Verification items for the finished model (mm, model axes). A direction names the side the tool comes from. Round coordinates to 2 decimals unless told otherwise and drop trailing zeros. Write each loop counter-clockwise with the first axis right and the second up, starting at its lowest first coordinate (ties: lowest second). Pieces come first, ordered by that corner, then holes. Notation, with made-up numbers: (78, -18.5) - (104, -18.5) arc R30 ccw to (104, 16.5) - close; hole circle Ø4 at (-26, 62.25). An arc over 180 degrees is marked (long way). Answer as a JSON object with one key per item and string values.
```python
from build123d import *

# Parameters (mm, degrees)
SKETCH1_W           = 144.53
SKETCH1_H           = 37.629508446
SKETCH1_R           = 1.6
BOSS_EXTRUDE1_DEPTH = 5


with BuildPart() as part:
    # Sketch1 → Boss-Extrude1 (new body)
    # profile 1 of 2: a face of its own
    with BuildSketch(Plane(origin=(0, 0, 0), x_dir=(1, 0, 0), z_dir=(0, 1, 0))):
        with Locations((-90.246144653, 26.488873013)):
            Rectangle(SKETCH1_W, SKETCH1_H)
        with Locations(Location((-77.511144653, 26.488627236, 0), (0, 0, 270))):
            Circle(SKETCH1_R, mode=Mode.SUBTRACT)
        with Locations(Location((-102.511144653, 26.488627236, 0), (0, 0, 270))):
            Circle(SKETCH1_R, mode=Mode.SUBTRACT)
        with Locations(Location((-127.511144653, 26.488627236, 0), (0, 0, 270))):
            Circle(SKETCH1_R, mode=Mode.SUBTRACT)
        with Locations(Location((-152.511144653, 26.488627236, 0), (0, 0, 270))):
            Circle(SKETCH1_R, mode=Mode.SUBTRACT)
    # profile 2 of 2: a face of its own
    with BuildSketch(Plane(origin=(0, 0, 0), x_dir=(1, 0, 0), z_dir=(0, 1, 0))):
        Polygon((28.788855347, 39.823627236), (23.318855347, 45.303627236), (-17.981144653, 45.303627236), (-17.981144653, 7.67411879), (19.408855347, 7.67411879), (28.788855347, 13.053627236), align=None)
        Polygon((20.478855347, 18.946495902), (13.563855347, 14.95411879), (6.648855347, 18.946495902), (6.648855347, 26.931250125), (13.563855347, 30.923627236), (20.478855347, 26.931250125), align=None, mode=Mode.SUBTRACT)
    extrude(amount=BOSS_EXTRUDE1_DEPTH)


solid = part.part
```
1. Cross-section at A-A (z = -22). Record the boundary of the cut face in (x, y), plus the area to 3 significant figures.
Completed:
{"outline": "(-162.51, 0) - (6.65, 0) - (6.65, 5) - (-162.51, 5) - close; (20.48, 0) - (28.79, 0) - (28.79, 5) - (20.48, 5) - close", "area": "887 mm^2"}
2. Access from +Z, -Z, +X, -X, +Y, -Y to the whole of each face (thin tool, end or side, straight path). Record for faces 1 (the face through (16.973, 2.465, -28.955)), 2 (the face through (28.789, 2, -26)).
Completed:
{"face 1": "+Y, -Y", "face 2": "+Z, -Z, +X, +Y, -Y"}
3. Go/stop test with a flat-tipped pin: pin 1 (1.9 mm diameter, centred on x = -127.51, z = -26.49, fed in from -Y). Record where the tip stops, or that it passes through.
Completed:
{"pin 1": "passes through"}
4. Cross-section at C-C (z = -10). Record the boundary of the cut face in (x, y).
Completed:
{"outline": "(-162.51, 0) - (23.46, 0) - (23.46, 5) - (-162.51, 5) - close"}
5. Material ranges on probe 1 along X at (y, z) = (1.3, -20.5); probe 2 along X at (y, z) = (3.85, -16); probe 3 along Z at (x, y) = (-126.5, 0.65), recorded low to high. Write a range as from..to.
Completed:
{"probe 1": "x = -162.51..6.65, 20.48..28.79", "probe 2": "x = -162.51..11.75, 15.38..28.79", "probe 3": "z = -45.3..-27.73, -25.25..-7.67"}
6. Cross-section at B-B (y = 2.85). Record the boundary of the cut face in (x, z).
Completed:
{"outline": "(-162.51, -45.3) - (23.32, -45.3) - (28.79, -39.82) - (28.79, -13.05) - (19.41, -7.67) - (-162.51, -7.67) - close; hole circle Ø3.2 at (-152.51, -26.49); hole circle Ø3.2 at (-127.51, -26.49); hole circle Ø3.2 at (-102.51, -26.49); hole circle Ø3.2 at (-77.51, -26.49); hole (6.65, -26.93) - (13.56, -30.92) - (20.48, -26.93) - (20.48, -18.95) - (13.56, -14.95) - (6.65, -18.95) - close"}
7. Mould release check, pull along Z, two halves, no side actions. Record for faces 3 (the face through (-129.073, 2.465, -26.835)), 4 (the face through (-100.925, 2.465, -26.697)), 5 (the face through (-68, 5, -27)), 6 (the face through (24.033, 2.465, -10.326)): released by +Z, released by -Z, zero draft, split by the parting line, or undercut.
Completed:
{"face 3": "undercut", "face 4": "undercut", "face 5": "zero draft", "face 6": "released by +Z"}
